from build123d import *

# Parameters (mm, degrees)
SALIENTE_EXTRUIR1_DEPTH = 9.66
CROQUIS2_R              = 3.98
SALIENTE_EXTRUIR2_DEPTH = 58.91
CORTAR_EXTRUIR1_REACH   = 80.623
CROQUIS3_R              = 2.6
CROQUIS4_R              = 5.075
CORTAR_EXTRUIR2_DEPTH   = 3.87


with BuildPart() as part:
    # Croquis1 → Saliente-Extruir1 (new body)
    with BuildSketch(Plane.XY):
        with BuildLine():
            Line((-29.715, 0), (29.715, 0))
            ThreePointArc((29.715, 0), (0, 24.43), (-29.715, 0))
        make_face()
    extrude(amount=-SALIENTE_EXTRUIR1_DEPTH)

    # Croquis2 → Saliente-Extruir2 (add)
    with BuildSketch(Plane(origin=(0, 0, -9.66), x_dir=(-1, 0, 0), z_dir=(0, 0, -1))):
        with Locations(Location((0, 12.215, 0), (0, 0, 180))):
            Circle(CROQUIS2_R)
    extrude(amount=SALIENTE_EXTRUIR2_DEPTH)

    # Croquis3 → Cortar-Extruir1 (cut, up to next)
    with BuildSketch(Plane.XY, mode=Mode.PRIVATE) as cortar_extruir1_sk1:
        with Locations((-14.334085257, 12.215)):
            Circle(CROQUIS3_R)
    cortar_extruir1_tool1 = extrude(cortar_extruir1_sk1.sketch, amount=-CORTAR_EXTRUIR1_REACH, mode=Mode.PRIVATE) & part.part
    # Croquis3 → Cortar-Extruir1 (cut, up to next)
    with BuildSketch(Plane.XY, mode=Mode.PRIVATE) as cortar_extruir1_sk2:
        with Locations((14.334085257, 12.215)):
            Circle(CROQUIS3_R)
    cortar_extruir1_tool2 = extrude(cortar_extruir1_sk2.sketch, amount=-CORTAR_EXTRUIR1_REACH, mode=Mode.PRIVATE) & part.part
    add(cortar_extruir1_tool1.solids().sort_by_distance((-14.334085, 12.215, 0))[0], mode=Mode.SUBTRACT)
    add(cortar_extruir1_tool2.solids().sort_by_distance((14.334085, 12.215, 0))[0], mode=Mode.SUBTRACT)

    # Croquis4 → Cortar-Extruir2 (cut)
    with BuildSketch(Plane.XY):
        with Locations((14.334085257, 12.215)):
            Circle(CROQUIS4_R)
        with Locations((-14.334085257, 12.215)):
            Circle(CROQUIS4_R)
    extrude(amount=-CORTAR_EXTRUIR2_DEPTH, mode=Mode.SUBTRACT)


solid = part.part
For this review, take the finished solid that the model builds, in its own axes (mm). A direction names the side the tool comes from. Round coordinates to 2 decimals unless told otherwise and drop trailing zeros. Order: outer loops, then holes, each group sorted by start corner. A loop starts at its lowest first (then second) coordinate and runs counter-clockwise, first axis right, second up. Notation, with made-up numbers: (2.5, 61.5) -> (56.5, 61.5) arc R21 ccw to (56.5, 94.5) -> close; hole circle Ø1 at (61, -15.75). An arc over 180 degrees is marked (long way). Write item = value, one per line. Start each with the question number.
1) Take a section at B-B on x = 0. State the section outline as (y, z) points (3 decimals), plus the area to 3 significant figures.
2) To check wall thickness, follow line 1 (Y direction, x = 1, z = -4); line 2 (Z direction, x = -10, y = 4.75); line 3 (Z direction, x = -12, y = 16). State the ranges of each line that lie inside material, in increasing order. Write a range as from..to.
3) Take a section at D-D on y = 19.25. State the section outline as (x, z) points.
4) Take a section at C-C on z = -7.5. State the section outline as (x, y) points (3 decimals), plus the area to 3 significant figures.
5) The part is to be moulded in two halves that separate along Y. For faces 1 (the face through (-0.86, 16.1, -38.7)), 2 (the face through (0.583, 24.424, -4.762)), 3 (the face through (-17, 13, -3.87)), say which applies: +Y half, -Y half, draft (parallel to the pull), parting line (faces both ways), or undercut.
6) Take a section at A-A on x = -16. State the section outline as (y, z) points, plus the area to 3 significant figures.
7) Insertion check: pin 1 (11.5 mm diameter, centred on x = -14.33, y = 12.22, fed in from -Z); pin 2 (3 mm diameter, centred on x = -16.5, y = 11.5, fed in from +Z); pin 3 (8 mm diameter, centred on y = 6.5, z = -55.5, fed in from +X). Each pin has a flat end and moves straight along its axis. Give the tip position at first contact, or say it passes through.
8) Tool access review of faces 4 (the face through (0, 10, 0)), 5 (the face through (13, 15, -3.87)): name each direction out of +Z, -Z, +X, -X, +Y, -Y from which nothing blocks a thin tool from reaching the whole face with its end or side.
Verdict:
q1.outline = (0, -9.66) -> (8.235, -9.66) -> (8.235, -68.57) -> (16.195, -68.57) -> (16.195, -9.66) -> (24.43, -9.66) -> (24.43, 0) -> (0, 0) -> close
q1.area = 705 mm2
q2.line_1 = 0..24.41
q2.line_2 = -9.66..0
q2.line_3 = -9.66..-3.87
q3.outline = (-16.94, -9.66) -> (16.94, -9.66) -> (16.94, 0) -> (-16.94, 0) -> close
q4.outline = (-29.715, 0) -> (29.715, 0) arc R30.287 ccw to start; hole circle Ø5.2 at (-14.334, 12.215); hole circle Ø5.2 at (14.334, 12.215)
q4.area = 1,050 mm2
q5.face_1 = parting line
q5.face_2 = +Y half
q5.face_3 = undercut
q6.outline = (0, -9.66) -> (10.22, -9.66) -> (10.22, -3.87) -> (7.42, -3.87) -> (7.42, 0) -> (0, 0) -> close; (14.21, -9.66) -> (19.86, -9.66) -> (19.86, 0) -> (17.01, 0) -> (17.01, -3.87) -> (14.21, -3.87) -> close
q6.area = 132 mm2
q7.pin_1 = -9.66
q7.pin_2 = -3.87
q7.pin_3 = 3.59
q8.face_4 = +Z, +X, -X, +Y, -Y
q8.face_5 = +Z
